Input: dimensioned drawing with shaded views. Units: mm. Origin: part minimum x, y, z. Coordinates: 2 decimals unless noted, no trailing zeros. Order: outer loops, then holes, each group sorted by start corner. A loop starts at its lowest first (then second) coordinate and runs counter-clockwise, first axis right, second up.
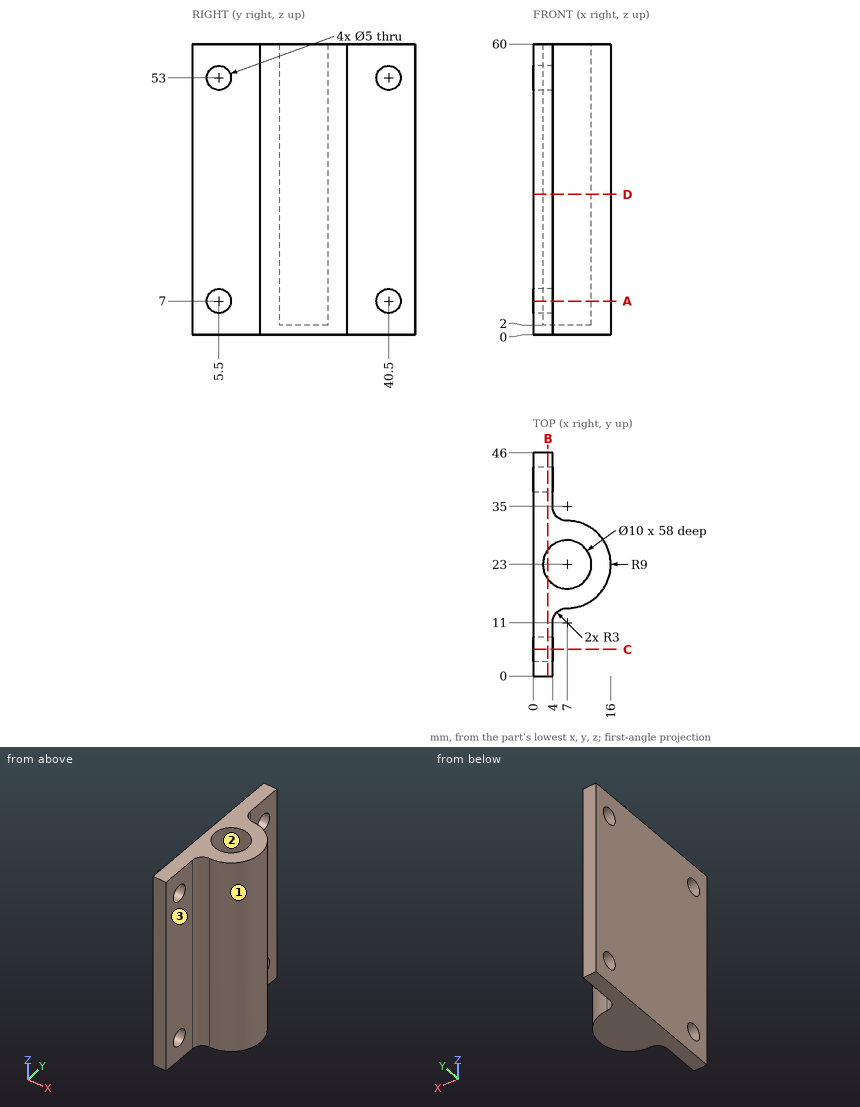
1. Section query C-C, the plane y = 5.5. Output: boundary loops of the cut face in (x, z), plus the area to 3 significant figures.
2. Section query B-B, the plane x = 3. Output: boundary loops of the cut face in (y, z).
3. Section query A-A, the plane z = 7. Output: boundary loops of the cut face in (x, y), plus the area to 3 significant figures.
4. Material intervals for line 1 along Z through (x, y) = (1.6, 40.5); line 2 along Z through (x, y) = (2.25, 41.5); line 3 along Y through (x, z) = (7, 17.5), sorted ascending.
5. Section query D-D, the plane z = 29. Output: boundary loops of the cut face in (x, y).
6. Contact query for flat-ended pins moving along their axis: P1, Ø9, axis at y = 39, z = 35.5, coming from the +X side; P2, Ø4.5, axis at y = 5.5, z = 53, coming from the +X side; P3, Ø1, axis at y = 33.5, z = 10.5, coming from the +X side. Output: stop coordinate, or through.
7. Draft query along Y for the marked faces 1, 2 and 3. Return one class per face: +Y half, -Y half, draft (parallel to the pull), parting line (faces both ways), or undercut.
Answer key:
1. outline: (0, 0) - (4, 0) - (4, 4.5) - (0, 4.5) - close; (0, 9.5) - (4, 9.5) - (4, 50.5) - (0, 50.5) - close; (0, 55.5) - (4, 55.5) - (4, 60) - (0, 60) - close
1. area: 200 mm2
2. outline: (0, 0) - (46, 0) - (46, 60) - (26, 60) - (26, 2) - (20, 2) - (20, 60) - (0, 60) - close; hole circle Ø5 at (5.5, 7); hole circle Ø5 at (5.5, 53); hole circle Ø5 at (40.5, 7); hole circle Ø5 at (40.5, 53)
3. outline: (0, 0) - (4, 0) - (4, 3) - (0, 3) - close; (0, 8) - (4, 8) - (4, 11) arc R3 cw to (7, 14) arc R9 ccw to (7, 32) arc R3 cw to (4, 35) - (4, 38) - (0, 38) - close; (0, 43) - (4, 43) - (4, 46) - (0, 46) - close; hole circle Ø10 at (7, 23)
3. area: 251 mm2
4. line 1: z = 0 to 4.5, 9.5 to 50.5, 55.5 to 60
4. line 2: z = 0 to 4.71, 9.29 to 50.71, 55.29 to 60
4. line 3: y = 14 to 18, 28 to 32
5. outline: (0, 0) - (4, 0) - (4, 11) arc R3 cw to (7, 14) arc R9 ccw to (7, 32) arc R3 cw to (4, 35) - (4, 46) - (0, 46) - close; hole circle Ø10 at (7, 23)
6. P1: stops at x = 4.04
6. P2: passes through
6. P3: stops at x = 4.76
7. face 1: parting line
7. face 2: undercut
7. face 3: draft
